Could you check a few things on this model? Use its own coordinates, in mm. Face numbers are marked on the shaded views. Coordinates: 2 decimals unless noted, no trailing zeros. Write each loop counter-clockwise with the first axis right and the second up, starting at its lowest first coordinate (ties: lowest second). Pieces come first, ordered by that corner, then holes.
```python
from build123d import *

# Parameters (mm, degrees)
SKETCH1_R           = 20
SKETCH1_R_2         = 2.1
BOSS_EXTRUDE1_DEPTH = 4.5
SKETCH2_R           = 1.6
CUT_EXTRUDE1_DEPTH  = 29.640006983
SKETCH5_R           = 3.5
CUT_EXTRUDE4_DEPTH  = 2
CIRPATTERN1_COUNT   = 6
SKETCH3_R           = 1.6
CUT_EXTRUDE2_DEPTH  = 29.640006983
SKETCH4_R           = 3.25
CUT_EXTRUDE3_DEPTH  = 2
CIRPATTERN2_COUNT   = 3


with BuildPart() as part:
    # Sketch1 → Boss-Extrude1 (new body)
    with BuildSketch(Plane(origin=(0, 0, 0), x_dir=(1, 0, 0), z_dir=(0, 1, 0))):
        with Locations(Location((0, 0, 0), (0, 0, 90))):
            Circle(SKETCH1_R)
        with Locations(Location((0, 0, 0), (0, 0, 90))):
            Circle(SKETCH1_R_2, mode=Mode.SUBTRACT)
    extrude(amount=BOSS_EXTRUDE1_DEPTH)

    # Sketch2 → Cut-Extrude1 (cut, through all)
    with BuildSketch(Plane.XZ):
        with Locations(Location((0, 16, 0), (0, 0, 270))):
            Circle(SKETCH2_R)
    cut_extrude1 = extrude(amount=-CUT_EXTRUDE1_DEPTH, mode=Mode.SUBTRACT)

    # Sketch5 → Cut-Extrude4 (cut)
    with BuildSketch(Plane(origin=(0, 4.5, 0), x_dir=(1, 0, 0), z_dir=(0, 1, 0))):
        with Locations(Location((0, -16, 0), (0, 0, 270))):
            Circle(SKETCH5_R)
    cut_extrude4 = extrude(amount=-CUT_EXTRUDE4_DEPTH, mode=Mode.SUBTRACT)

    # CirPattern1: Cut-Extrude1, Cut-Extrude4 ×6 about axis
    cirpattern1_axis = Axis((0, 0, 0), (0, 1, 0))
    add([cut_extrude1.rotate(cirpattern1_axis, i * 360 / CIRPATTERN1_COUNT) for i in range(1, CIRPATTERN1_COUNT)], mode=Mode.SUBTRACT)
    add([cut_extrude4.rotate(cirpattern1_axis, i * 360 / CIRPATTERN1_COUNT) for i in range(1, CIRPATTERN1_COUNT)], mode=Mode.SUBTRACT)

    # Sketch3 → Cut-Extrude2 (cut, through all)
    with BuildSketch(Plane(origin=(0, 4.5, 0), x_dir=(1, 0, 0), z_dir=(0, 1, 0))):
        with Locations(Location((0, 6.5, 0), (0, 0, 270))):
            Circle(SKETCH3_R)
    cut_extrude2 = extrude(amount=-CUT_EXTRUDE2_DEPTH, mode=Mode.SUBTRACT)

    # Sketch4 → Cut-Extrude3 (cut)
    with BuildSketch(Plane(origin=(0, 4.5, 0), x_dir=(1, 0, 0), z_dir=(0, 1, 0))):
        with Locations(Location((0, 6.5, 0), (0, 0, 270))):
            Circle(SKETCH4_R)
    cut_extrude3 = extrude(amount=-CUT_EXTRUDE3_DEPTH, mode=Mode.SUBTRACT)

    # CirPattern2: Cut-Extrude2, Cut-Extrude3 ×3 about axis
    cirpattern2_axis = Axis((0, 0, 0), (0, 1, 0))
    add([cut_extrude2.rotate(cirpattern2_axis, i * 360 / CIRPATTERN2_COUNT) for i in range(1, CIRPATTERN2_COUNT)], mode=Mode.SUBTRACT)
    add([cut_extrude3.rotate(cirpattern2_axis, i * 360 / CIRPATTERN2_COUNT) for i in range(1, CIRPATTERN2_COUNT)], mode=Mode.SUBTRACT)


solid = part.part
```
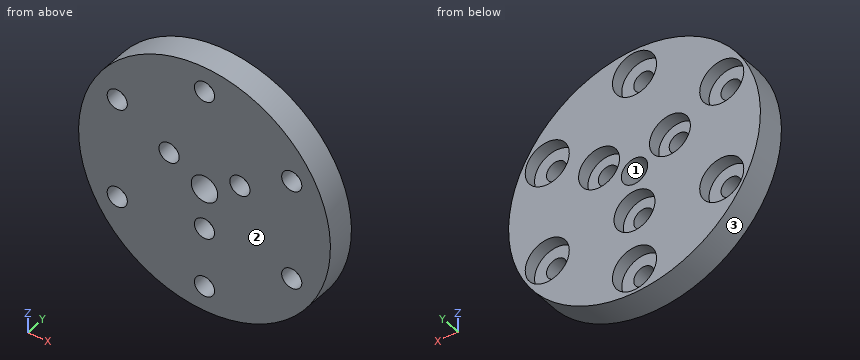
1. Please list where these lines run through material, in increasing order: line 1 along Z through (x, y) = (-11.5, 3.75); line 2 along Z through (x, y) = (16.5, 3.45); line 3 along Y through (x, z) = (12, -9.5).
Verdict:
line 1: z = -16.36 to -10.59, -5.41 to 5.41, 10.59 to 16.36
line 2: z = -11.3 to -10.29, -5.71 to 5.71, 10.29 to 11.3
line 3: y = 0 to 2.5
2. If we mould it in two halves opening along Z, with no side actions, what happens to the marked faces 1, 2 and 3? For each: pulls with the +Z half, pulls with the -Z half, needs draft (parallel to the pull), parting line crosses it, or undercut.
Verdict:
face 1: undercut
face 2: needs draft
face 3: parting line crosses it
3. I want a section at B-B on z = -16. Please give me the cut outline in (x, y).
Verdict:
outline: (-12, 0) - (-1.6, 0) - (-1.6, 2.5) - (-3.5, 2.5) - (-3.5, 4.5) - (-12, 4.5) - close; (1.6, 0) - (12, 0) - (12, 4.5) - (3.5, 4.5) - (3.5, 2.5) - (1.6, 2.5) - close
4. For pin 1 (3 mm diameter, centred on x = -5, z = 4.5, fed in from +Y); pin 2 (2 mm diameter, centred on y = 3, z = 7, fed in from +X); pin 3 (8 mm diameter, centred on x = 0, z = -16, fed in from +Y), each with a flat end and sliding along its axis, tell me the tip position at first contact or that it passes through.
Verdict:
pin 1: stops at y = 2.5
pin 2: stops at x = 19.08
pin 3: stops at y = 4.5
5. I want a section at D-D on z = 8. Please give me the cut outline in (x, y), plus the area to 3 significant figures.
Verdict:
outline: (-18.33, 0) - (-15.46, 0) - (-15.46, 2.5) - (-17.36, 2.5) - (-17.36, 4.5) - (-18.33, 4.5) - close; (-12.26, 0) - (12.26, 0) - (12.26, 2.5) - (10.36, 2.5) - (10.36, 4.5) - (-10.36, 4.5) - (-10.36, 2.5) - (-12.26, 2.5) - close; (15.46, 0) - (18.33, 0) - (18.33, 4.5) - (17.36, 4.5) - (17.36, 2.5) - (15.46, 2.5) - close
area: 121 mm2
6. I want a section at A-A on x = 0. Give the number of separate pieces and of enclosed holes in the cut face, plus the area to 3 significant figures.
Verdict:
separate pieces: 5
enclosed holes: 0
area: 96.1 mm2
